from build123d import *

# Parameters (mm, degrees)
F0_W     = 50
F0_H     = 50
F1_DEPTH = 50
F2_R     = 12.5
F3_DEPTH = 50.001
F4_R     = 5


with BuildPart() as f1:
    # F0 (on Top) → F1 (new body)
    with BuildSketch(Plane.XY):
        with Locations((25, 25)):
            Rectangle(F0_W, F0_H)
    extrude(amount=F1_DEPTH)

    # F2 (on face) → F3 (cut, through all)
    with BuildSketch(Plane.XZ):
        with Locations((25, 25)):
            Circle(F2_R)
    extrude(amount=-F3_DEPTH, mode=Mode.SUBTRACT)

    # F4
    f4_edges = [f1.edges().sort_by_distance(p)[0] for p in [
        (25, 0, 50),
        (50, 25, 50),
        (50, 0, 25),
    ]]
    fillet(f4_edges, radius=F4_R)


solid = f1.part
Source: CAD feature listing. Evaluate the final solid. Frame: model axes, mm. Give positions to 0.01 mm unless a question says otherwise; leave off trailing zeros. Write each loop counter-clockwise with the first axis right and the second up, starting at its lowest first coordinate (ties: lowest second). Pieces come first, ordered by that corner, then holes. Notation, with made-up numbers: (35, 26) - (60, 26) arc R12 ccw to (60, 44) - close; hole circle Ø5 at (85.5, 60). An arc over 180 degrees is marked (long way). Write item = value, one per line. Start each with the question number.
Q1. Material intervals for probe 1 along Z at (x, y) = (25, 13); probe 2 along Z at (x, y) = (29.5, 5); probe 3 along X at (y, z) = (12, 23), sorted ascending.
Q2. Cut plane A-A, the plane z = 25. Return loops of the section in (x, y).
Q3. Cut plane B-B, the plane x = 20. Return loops of the section in (y, z), then the cut area to 3 significant figures.
Q4. Draft query along X for faces 1 (the flat face through (50, 27, 22)), 2 (the cylindrical face through (15.08, 24.65, 17.394)), 3 (the flat face through (0, 25, 25)), 4 (the cylindrical face through (23, 1, 48)). Return one class per face: +X half, -X half, draft (parallel to the pull), parting line (faces both ways), or undercut.
Q5. Pin query (flat end, axial travel): pin 1 Ø15 at (x, z) = (25, 25) entering from +Y. Return the tip coordinate at first contact, or that it passes through.
Q6. Cut plane C-C, the plane y = 39. Return loops of the section in (x, z), then the cut area to 3 significant figures.
Computed values:
q1.probe_1 = 0 to 12.5, 37.5 to 50
q1.probe_2 = 0 to 13.34, 36.66 to 50
q1.probe_3 = 0 to 12.66, 37.34 to 50
q2.outline = (0, 0) - (12.5, 0) - (12.5, 50) - (0, 50) - close; (37.5, 0) - (45, 0) arc R5 ccw to (50, 5) - (50, 50) - (37.5, 50) - close
q3.outline = (0, 0) - (50, 0) - (50, 13.54) - (0, 13.54) - close; (0, 36.46) - (50, 36.46) - (50, 50) - (5, 50) arc R5 ccw to (0, 45) - close
q3.area = 1,350 mm²
q4.face_1 = +X half
q4.face_2 = undercut
q4.face_3 = -X half
q4.face_4 = draft
q5.pin_1 = through
q6.outline = (0, 0) - (50, 0) - (50, 45) arc R5 ccw to (45, 50) - (0, 50) - close; hole circle Ø25 at (25, 25)
q6.area = 2,000 mm²
